```python
from build123d import *

# Parameters (mm, degrees)
SCHIZZO1_R                   = 3
ESTRUSIONE_ESTRUSIONE1_DEPTH = 1
SCHIZZO2_R                   = 2.5
ESTRUSIONE_ESTRUSIONE2_DEPTH = 7.6
RACCORDO3_R                  = 2
SCHIZZO6_R                   = 0.5
SCHIZZO7_W                   = 4.951519697
SCHIZZO7_H                   = 4.598065652
TAGLIO_ESTRUSIONE1_DEPTH     = 10


with BuildPart() as part:
    # Schizzo1 → Estrusione-Estrusione1 (new body)
    with BuildSketch(Plane(origin=(0, 0, 0), x_dir=(1, 0, 0), z_dir=(0, 1, 0))):
        with Locations(Location((0, 0, 0), (0, 0, 270))):
            Circle(SCHIZZO1_R)
    extrude(amount=ESTRUSIONE_ESTRUSIONE1_DEPTH)

    # Schizzo2 → Estrusione-Estrusione2 (add)
    with BuildSketch(Plane(origin=(0, 1, 0), x_dir=(1, 0, 0), z_dir=(0, 1, 0))):
        with Locations(Location((0, 0, 0), (0, 0, 90))):
            Circle(SCHIZZO2_R)
    extrude(amount=ESTRUSIONE_ESTRUSIONE2_DEPTH)

    # Raccordo3
    raccordo3_edges = [part.edges().sort_by_distance(p)[0] for p in [
        (0, 8.6, 2.5),
    ]]
    fillet(raccordo3_edges, radius=RACCORDO3_R)

    # Sweep1: sweep along a path in Schizzo5
    with BuildLine(Plane(origin=(1.27, 0, 0), x_dir=(0, 0, -1), z_dir=(1, 0, 0))) as sweep1_path:
        Line((0, 0), (0, -2.5))
        Line((0, -2.5), (2, -2.5))
        Line((2, -2.5), (2, -8.5))
    # Schizzo6 → Sweep1 (sweep)
    with BuildSketch(Plane.XZ):
        with Locations((1.27, -0.022402078)):
            Circle(SCHIZZO6_R)
    sweep1 = sweep(path=sweep1_path.line, transition=Transition.RIGHT)

    # Specchia1: Sweep1 across plane
    add(sweep1.mirror(Plane(origin=(0, 0, 0), x_dir=(0, 0, 1), z_dir=(1, 0, 0))))

    # Schizzo7 → Taglio-Estrusione1 (cut)
    with BuildSketch(Plane(origin=(2.5, 0, 0), x_dir=(0, 0, -1), z_dir=(1, 0, 0))):
        with Locations((0.024240151, 0.648217725)):
            Rectangle(SCHIZZO7_W, SCHIZZO7_H)
    extrude(amount=TAGLIO_ESTRUSIONE1_DEPTH, mode=Mode.SUBTRACT)


solid = part.part
```
CAD build for the part. Positions are in the model's coordinates, mm. A direction names the side the tool comes from. Round coordinates to 2 decimals unless told otherwise and drop trailing zeros. Loops run counter-clockwise (first coordinate to the right, second up) from the corner with the lowest first, then second, coordinate; pieces in that order, holes last. Notation, with made-up numbers: (54.5, 77.5) - (111.5, 77.5) arc R20 cw to (111.5, 94.5) - close; hole circle Ø3 at (58, 39.5). An arc over 180 degrees is marked (long way). Return JSON: item names as keys, results as strings. Group by question number.
Q1. Band-saw the part on A-A on y = 3.5. Give the cut face in (x, z).
Q2. Flat gauge pin, fed straight in: pin 1 Ø1 at (y, z) = (-5, -2) entering from +X. Where does the tip first touch, or does it go through?
Q3. Drill centre lines: line 1 along Y through (x, z) = (-1.35, -2.25); line 2 along Y through (x, z) = (1.9, -1.9); line 3 along Y through (x, z) = (-1.6, -2.05). Where is each one in solid material? Low to high. Write a range as [from, to].
Q4. Tool access for faces 4 (the face through (-1.501, -5.284, -2.466)), 5 (the face through (-2, 1, 2)), 6 (the face through (1.205, -1.179, 0.473)): list every direction of +Z, -Z, +X, -X, +Y, -Y with a clear straight run to the whole face (end or side of a thin tool).
Q5. Band-saw the part on B-B on y = -3.5. Give the cut face in (x, z), plus the area to 3 significant figures.
Q6. Two-plate mould, pull along X, no slides. Class faces 1 (the face through (-3, 0.5, -0.1)), 2 (the face through (1, -8.5, -2)), 3 (the face through (-1.732, -2.286, -1.043)): +X half, -X half, draft (parallel to the pull), parting line (faces both ways), or undercut.
Q7. Band-saw the part on C-C on y = 0.75. Give the cut face in (x, z), plus the area to 3 significant figures.
Solutions:
{
 "1": {"outline": "circle Ø5 at (0, 0)"},
 "2": {"pin 1": "stops at x = 1.77"},
 "3": {"line 1": "y = [-8.5, -1.98], [0, 1]", "line 2": "y = [0, 1]", "line 3": "y = [-8.5, -2.1], [0, 1]"},
 "4": {"face 4": "-Y", "face 5": "+Y", "face 6": "none"},
 "5": {"outline": "circle Ø1 at (-1.27, -2.02); circle Ø1 at (1.27, -2.02)", "area": "1.57 mm^2"},
 "6": {"face 1": "parting line", "face 2": "draft", "face 3": "undercut"},
 "7": {"outline": "(2.5, -1.66) - (2.5, 1.66) arc R3 ccw (long way) to start", "area": "27.1 mm^2"}
}
